Autodesk Inventor part; units mm, degrees
ref_plane "YZ Plane" through (0, 0, 0) normal (1, 0, 0) x (0, 1, 0)
ref_plane "XZ Plane" through (0, 0, 0) normal (0, 1, 0) x (-1, 0, 0)
ref_plane "XY Plane" through (0, 0, 0) normal (0, 0, 1) x (1, 0, 0)
sketch "Sketch2" plane through (0, 0, 0) normal (0, 0, 1) x (-1, 0, 0)
  line L0 (0, -22.8) -> (0, 136.8) construction
  line L1 (0, 114) -> (-92.5, 114)
  line L2 (-92.5, 114) -> (-92.5, 109)
  line L3 (-92.5, 109) -> (-81.5, 109)
  line L4 (-81.5, 109) -> (-81.5, 0)
  line L5 (-81.5, 0) -> (-72.5, 0)
  line L6 (-72.5, 0) -> (-72.5, 110)
  line L7 (-72.5, 110) -> (0, 110)
  line L8 (0, 114) -> (0, 110)
  line L9 (18.5, 0) -> (-111, 0) construction
  point P0 (0, 0)
  dimension "d4" = 5
  dimension "d5" = 11
  dimension "d6" = 9
  dimension "d8" = 110
  dimension "d9" = 4
  dimension "d38" = 81.5
revolve "Revolution1" add sketch "Sketch2" angle 360 about axis through (0, 0, 0) along (0, -1, 0)
sketch "Sketch3" plane through (0, -109, 0) normal (0, 1, 0) x (1, 0, 0)
  line L0 (0, 129.5) -> (0, -129.5) construction
  line L1 (129.5, 0) -> (-129.5, 0) construction
  circle A0 centre (0, 0) radius 87 construction
  circle A1 centre (0, 0) radius 81.5 construction
  circle A2 centre (0, 0) radius 92.5 construction
  point P0 (0, 87)
  dimension "d11" = 5.5
  dimension "d12" = 5.5
hole "Hole1" at (0, -109, -87) direction (0, -1, 0) diameter 4.5 end through all
pattern_circular "Circular Pattern1" count 5 over 360 about axis through (0, -10, 0) along (0, 1, 0) of "Hole1"
sketch "Sketch5" plane through (0, 0, 0) normal (0, 1, 0) x (1, 0, 0)
  line L0 (0, 129.5) -> (0, -129.5) construction
  line L1 (129.5, 0) -> (-129.5, 0) construction
  circle A0 centre (0, 0) radius 77 construction
  circle A1 centre (0, 0) radius 72.5 construction
  circle A2 centre (0, 0) radius 81.5 construction
  point P0 (0, 77)
  point P1 (-66.684, 38.5)
  point P2 (-66.684, -38.5)
  point P3 (0, -77)
  point P4 (66.684, -38.5)
  point P5 (66.684, 38.5)
  dimension "d39" = 4.5
  dimension "d40" = 4.5
  dimension "d43" = 360
hole "Hole2" at (0, 0, -77) at (-66.684, 0, -38.5) at (-66.684, 0, 38.5) at (0, 0, 77) at (66.684, 0, 38.5) at (66.684, 0, -38.5) direction (0, -1, 0) diameter 3.242 depth 13 tip angle 118
equation "\"d11\" = d12"
equation "\"d39\" = d40"
properties part number "Base" material "Aluminum 6061"
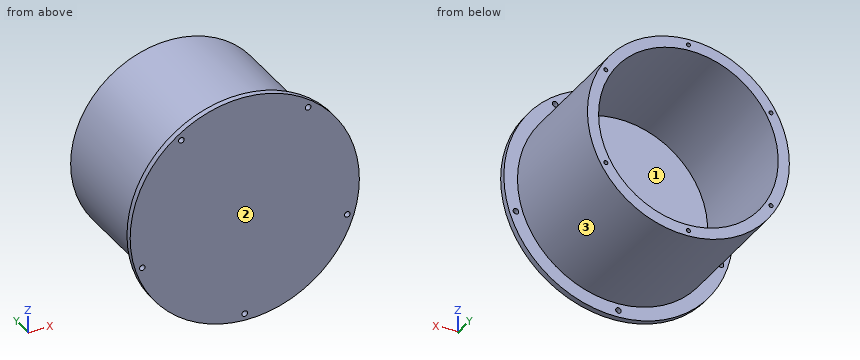
Source: CAD feature listing. Evaluate the final solid. Frame: model axes, mm. Face numbers are marked on the shaded views. Give positions to 0.01 mm unless a question says otherwise; leave off trailing zeros. Loops run counter-clockwise (first coordinate to the right, second up) from the corner with the lowest first, then second, coordinate; pieces in that order, holes last. Notation, with made-up numbers: (15, 81.5) -> (45, 81.5) arc R7 cw to (45, 88.5) -> close; hole circle Ø7 at (5.5, -2). An arc over 180 degrees is marked (long way). Use a Markdown table: item, result. Add a question column.
1) Section query D-D, the plane z = 48. Return the cut outline in (x, y), then the cut area to 3 significant figures.
2) Section query A-A, the plane z = 0. Return the cut outline in (x, y).
3) Section query B-B, the plane y = -80. Return the cut outline in (x, z), then the cut area to 3 significant figures.
4) First-contact query: pin 1 (3.5 mm diameter, centred on x = 0, z = -87, fed in from -Y); pin 2 (5 mm diameter, centred on x = 12, z = -6.5, fed in from +Y); pin 3 (3 mm diameter, centred on y = -25, z = -29.5, fed in from -X); pin 4 (10 mm diameter, centred on y = -44, z = 67, fed in from -X). Flat tips, straight axial feed; report the tip coordinate or a pass-through.
5) Line query: line 1 along Z through (x, y) = (0, -5); line 2 along X through (y, z) = (-69, 1); line 3 along Z through (x, y) = (0, -81.5). Output: solid intervals per line, ascending. Write a range as [from, to].
6) Section query C-C, the plane x = -76. Return the cut outline in (y, z).
7) Pull-direction query (X, two-part tool) for the marked faces 1, 2 and 3; classes: +X half, -X half, draft (parallel to the pull), parting line (faces both ways), or undercut.
Numbers:
| question | item | result |
|---|---|---|
| 1 | outline | (-79.07, -114) -> (79.07, -114) -> (79.07, -109) -> (65.87, -109) -> (65.87, 0) -> (54.33, 0) -> (54.33, -110) -> (-54.33, -110) -> (-54.33, 0) -> (-65.87, 0) -> (-65.87, -109) -> (-79.07, -109) -> close |
| 1 | area | 3,200 mm2 |
| 2 | outline | (-92.5, -114) -> (92.5, -114) -> (92.5, -109) -> (81.5, -109) -> (81.5, 0) -> (72.5, 0) -> (72.5, -110) -> (-72.5, -110) -> (-72.5, 0) -> (-81.5, 0) -> (-81.5, -109) -> (-92.5, -109) -> close |
| 3 | outline | circle Ø163 at (0, 0); hole circle Ø145 at (0, 0) |
| 3 | area | 4,350 mm2 |
| 4 | pin 1 | passes through |
| 4 | pin 2 | stops at y = -110 |
| 4 | pin 3 | stops at x = -76.54 |
| 4 | pin 4 | stops at x = -52.9 |
| 5 | line 1 | z = [-81.5, -78.62], [-75.38, -72.5], [72.5, 75.38], [78.62, 81.5] |
| 5 | line 2 | x = [-81.49, -72.49], [72.49, 81.49] |
| 5 | line 3 | z = [-81.5, -72.5], [72.5, 81.5] |
| 6 | outline | (-114, -52.73) -> (-109, -52.73) -> (-109, -29.43) -> (0, -29.43) -> (0, 29.43) -> (-109, 29.43) -> (-109, 52.73) -> (-114, 52.73) -> close |
| 7 | face 1 | undercut |
| 7 | face 2 | draft |
| 7 | face 3 | parting line |
